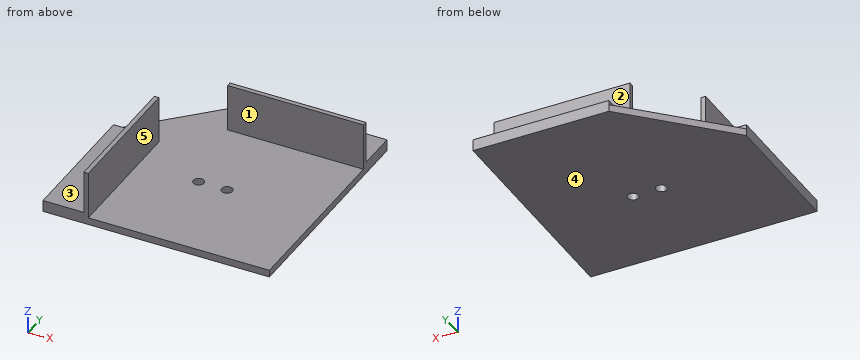
```python
from build123d import *

# Parameters (mm, degrees)
F1_DEPTH  = 8
F2_W      = 152.4
F2_H      = 50.8
F2_W_2    = 50.8
F2_H_2    = 152.4
F3_DEPTH  = 5
F5_W      = 152.4
F5_H      = 5
F6_DEPTH  = 48.26
F7_R      = 6
F8_DEPTH  = 8
F9_R      = 6
F10_DEPTH = 8
F4_W      = 5
F4_H      = 152.4
F11_DEPTH = 48.26


with BuildPart() as f1:
    # F0 (on Top) → F1 (new body)
    with BuildSketch(Plane.XY):
        Polygon((-10.222614, 146.12082), (-111.822614, 44.52082), (-111.822614, -107.87918), (142.177386, -107.87918), (142.177386, 146.12082), align=None)
    extrude(amount=F1_DEPTH)

    # F2 (on face) → F3 (join)
    with BuildSketch(Plane.XY.offset(8)):
        with Locations((65.977386, 120.72082)):
            Rectangle(F2_W, F2_H)
        with Locations((-86.422614, -31.67918)):
            Rectangle(F2_W_2, F2_H_2)
    extrude(amount=F3_DEPTH)

    # F5 (on face) → F6 (join)
    with BuildSketch(Plane.XY.offset(13)):
        with Locations((65.977386, 97.82082)):
            Rectangle(F5_W, F5_H)
    extrude(amount=F6_DEPTH)

    # F7 (on face) → F8 (cut)
    with BuildSketch(Plane.XY.offset(8)):
        with Locations((6.839792, 0)):
            Circle(F7_R)
    extrude(amount=-F8_DEPTH, mode=Mode.SUBTRACT)

    # F9 (on face) → F10 (cut)
    with BuildSketch(Plane.XY.offset(8)):
        with Locations((38.607758, 0)):
            Circle(F9_R)
    extrude(amount=-F10_DEPTH, mode=Mode.SUBTRACT)

    # F4 (on face) → F11 (join)
    with BuildSketch(Plane.XY.offset(13)):
        with Locations((-63.522614, -31.67918)):
            Rectangle(F4_W, F4_H)
    extrude(amount=F11_DEPTH)


solid = f1.part
```
Input: part model. Units: mm. Frame: model coordinates. Face numbers are marked on the shaded views. A direction names the side the tool comes from. Coordinates: 2 decimals unless noted, no trailing zeros. Write each loop counter-clockwise with the first axis right and the second up, starting at its lowest first coordinate (ties: lowest second). Pieces come first, ordered by that corner, then holes. Notation, with made-up numbers: (38.25, 20.5) -> (79.25, 20.5) arc R33 cw to (79.25, 51.5) -> close; hole circle Ø8 at (79, -23.5). An arc over 180 degrees is marked (long way). Answer as a JSON object with one key per item and string values.
1. Access query for the marked faces 1, 2 and 3. Directions: +Z, -Z, +X, -X, +Y, -Y. A direction counts if a zero-diameter tool reaches every point of the face in a straight line with its end or side. Return the directions, or none.
Result set:
{"face 1": "+Z, +X, -X, -Y", "face 2": "+Z, +X, -X, +Y", "face 3": "+Z, -X, +Y, -Y"}
2. Mould query, pull axis X, two halves, no side actions, for the marked faces 4 and 5. Classes: released by +X, released by -X, zero draft, split by the parting line, or undercut.
Result set:
{"face 4": "zero draft", "face 5": "released by +X"}
3. Material intervals for line 1 (X direction, y = -3, z = 4.5); line 2 (Z direction, x = 13.5, y = 37); line 3 (Y direction, x = 110, z = 15), sorted ascending. Write a range as from..to.
Result set:
{"line 1": "x = -111.82..1.64, 12.04..33.41, 43.8..142.18", "line 2": "z = 0..8", "line 3": "y = 95.32..100.32"}
4. First-contact query: P1, Ø12, axis at x = -30, y = 9, coming from the -Z side; P2, Ø12, axis at y = -39, z = 54, coming from the -X side; P3, Ø14.5, axis at x = 63, z = 38.5, coming from the +Y side; P4, Ø5, axis at x = 26, y = -38.5, coming from the +Z side. Flat tips, straight axial feed; report the tip coordinate or a pass-through.
Result set:
{"P1": "stops at z = 0", "P2": "stops at x = -66.02", "P3": "stops at y = 100.32", "P4": "stops at z = 8"}
5. Section B-B on y = 0. Return the cut outline in (x, z), then the cut area to 3 significant figures.
Result set:
{"outline": "(-111.82, 0) -> (0.84, 0) -> (0.84, 8) -> (-61.02, 8) -> (-61.02, 61.26) -> (-66.02, 61.26) -> (-66.02, 13) -> (-111.82, 13) -> close; (12.84, 0) -> (32.61, 0) -> (32.61, 8) -> (12.84, 8) -> close; (44.61, 0) -> (142.18, 0) -> (142.18, 8) -> (44.61, 8) -> close", "area": "2,340 mm2"}
6. Section C-C on x = 82. Return the cut outline in (y, z), then the cut area to 3 significant figures.
Result set:
{"outline": "(-107.88, 0) -> (146.12, 0) -> (146.12, 13) -> (100.32, 13) -> (100.32, 61.26) -> (95.32, 61.26) -> (95.32, 8) -> (-107.88, 8) -> close", "area": "2,530 mm2"}
7. Section A-A on z = 55.5. Return the cut outline in (x, y).
Result set:
{"outline": "(-66.02, -107.88) -> (-61.02, -107.88) -> (-61.02, 44.52) -> (-66.02, 44.52) -> close; (-10.22, 95.32) -> (142.18, 95.32) -> (142.18, 100.32) -> (-10.22, 100.32) -> close"}
8. Section D-D on y = 32. Return the cut outline in (x, z), then the cut area to 3 significant figures.
Result set:
{"outline": "(-111.82, 0) -> (142.18, 0) -> (142.18, 8) -> (-61.02, 8) -> (-61.02, 61.26) -> (-66.02, 61.26) -> (-66.02, 13) -> (-111.82, 13) -> close", "area": "2,530 mm2"}
